```python
from build123d import *

# Parameters (mm, degrees)
ESQUISSE3_R             = 23.853720884
ENL_V_MAT_EXTRU_2_DEPTH = 6
ESQUISSE4_W             = 60
ESQUISSE4_H             = 84
ENL_V_MAT_EXTRU_3_DEPTH = 42.231056353


with BuildPart() as part:
    # Esquisse1 → Base-Révolution (revolve)
    with BuildSketch(Plane.XY):
        with BuildLine():
            Line((0, 12), (0, 20))
            Line((0, 20), (4, 20))
            ThreePointArc((4, 20), (6, 18), (8, 20))
            Line((8, 20), (29, 20))
            Line((29, 20), (30, 19))
            Line((30, 19), (30, 16))
            Line((30, 16), (28, 14))
            Line((28, 14), (22, 14))
            Line((22, 14), (22, 12))
            Line((22, 12), (0, 12))
        make_face()
    revolve(axis=Axis((-10, 0, 0), (1, 0, 0)))

    # Esquisse3 → Enlèv. mat.-Extru.2 (cut)
    with BuildSketch(Plane.ZY):
        Circle(ESQUISSE3_R)
        Polygon((-20.732050808, 0), (-10.366025404, 17.954482672), (10.366025404, 17.954482672), (20.732050808, 0), (10.366025404, -17.954482672), (-10.366025404, -17.954482672), align=None, mode=Mode.SUBTRACT)
    extrude(amount=-ENL_V_MAT_EXTRU_2_DEPTH, mode=Mode.SUBTRACT)

    # Esquisse4 → Enlèv. mat.-Extru.3 (cut, through all)
    with BuildSketch(Plane(origin=(0, 0, 0), x_dir=(1, 0, 0), z_dir=(0, 1, 0))):
        with Locations((20, -4)):
            Rectangle(ESQUISSE4_W, ESQUISSE4_H)
    extrude(amount=-ENL_V_MAT_EXTRU_3_DEPTH, mode=Mode.SUBTRACT)


solid = part.part
```
Read the model definition and answer for the solid it produces. Units are mm, in the model's axes. A direction names the side the tool comes from. Give positions to 0.01 mm unless a question says otherwise; leave off trailing zeros. Order: outer loops, then holes, each group sorted by start corner. A loop starts at its lowest first (then second) coordinate and runs counter-clockwise, first axis right, second up.
(1) Given pin 1 (1 mm diameter, centred on y = 9, z = 15.5, fed in from -X); pin 2 (6.5 mm diameter, centred on x = 2, z = -2, fed in from +Y); pin 3 (3 mm diameter, centred on x = 23.5, y = 13, fed in from +Z); pin 4 (1.5 mm diameter, centred on x = 16, y = 7, fed in from -Z), each flat-ended and moving along its own axis, determine where each tip first touches the part or whether it passes through.
(2) Find section A-A (z = 0). Give the vertices of the cut face in (x, y), plus the area to 3 significant figures.
(3) For a pull along Z with two mould halves and no side action, classify faces 6 (the conical face through (28.319, 14.316, -0.315)), 7 (the flat face through (2.29, 9.08, 15.49)), 8 (the cylindrical face through (11, 12, 0)), 9 (the cylindrical face through (19, 20, 0)) as released by +Z, released by -Z, zero draft, split by the parting line, or undercut.
(4) Find section B-B (x = 12). Give the vertices of the cut face in (y, z), plus the area to 3 significant figures.
(5) For faces 1 (the flat face through (2, 17.954, 0)), 2 (the flat face through (15, 0, -16)), 3 (the cylindrical face through (2.03, 0.68, 19.99)), 4 (the flat face through (2.29, 8.87, -15.61)), 5 (the flat face through (22, 12.2, 0.1)), determine the directions among +Z, -Z, +X, -X, +Y, -Y from which every point of the face is accessible in a straight line to the end or side of a thin tool.
(6) Straight lines are drawn through the part: L1, parallel to Z at x = 7.5, y = 4.75; L2, parallel to Z at x = 26, y = 8.75; L3, parallel to X at y = 12.25, z = -4.5. For each, find the intervals that lie inside material, in ascending order.
Result sheet:
1. pin 1: stops at x = 0
1. pin 2: stops at y = 17.95
1. pin 3: stops at z = 16.36
1. pin 4: stops at z = -19
2. outline: (0, 12) - (22, 12) - (22, 14) - (28, 14) - (30, 16) - (30, 19) - (29, 20) - (8, 20) arc R2 cw to (6, 18) - (6, 17.95) - (0, 17.95) - close
2. area: 206 mm2
3. face 6: undercut
3. face 7: released by +Z
3. face 8: undercut
3. face 9: split by the parting line
4. outline: (0, -20) arc R20 ccw to (0, 20) - (0, 12) arc R12 cw to (0, -12) - close
4. area: 402 mm2
5. face 1: +Z, -Z, -X, +Y
5. face 2: +Z, -Z, +X, -X, -Y
5. face 3: +Z, +X, -X, +Y
5. face 4: -Z, -X, +Y
5. face 5: +X, -Y
6. L1: z = -18.06 to -11.02, 11.02 to 18.06
6. L2: z = -17.98 to -10.93, 10.93 to 17.98
6. L3: x = 0 to 22
